Job drawing, mm, ordinate dimensions from the low corner. One solid piece. A direction names the side the tool comes from. Give positions to 0.01 mm unless a question says otherwise; leave off trailing zeros. Loops run counter-clockwise (first coordinate to the right, second up) from the corner with the lowest first, then second, coordinate; pieces in that order, holes last.
Item 1: Saw through at B-B on z = 1.5. Give the cut face in (x, y), plus the area to 3 significant figures.
Item 2: Mould opens along X. For the marked faces 5, 6, 7 and 8 say: released by +X, released by -X, zero draft, split by the parting line, or undercut.
Item 3: Drop flat-ended pins along their axis: P1, Ø0.8, axis at x = 12, z = 4, coming from the +Y side; P2, Ø8, axis at x = 8, y = 9, coming from the -Z side; P3, Ø0.5, axis at x = 12.5, y = 16, coming from the +Z side; P4, Ø4, axis at x = 7.5, y = 7.5, coming from the +Z side. Give the stop position or say it passes through.
Item 4: Saw through at A-A on x = 7.5. Give the cut face in (y, z).
Item 5: Probe probe 1 along Y at (x, z) = (7.5, 3.75); probe 2 along Z at (x, y) = (11.5, 6); probe 3 along Z at (x, y) = (11.5, 17.25). List the from-to ranges inside material, lowest first.
Item 6: Saw through at D-D on y = 13. Give the cut face in (x, z), plus the area to 3 significant figures.
Item 7: Which spindle directions (+Z, -Z, +X, -X, +Y, -Y) get a long thin tool onto all of the face, cutting with end or side? Do the marked faces 1, 2, 3 and 4. Say none if no direction does.
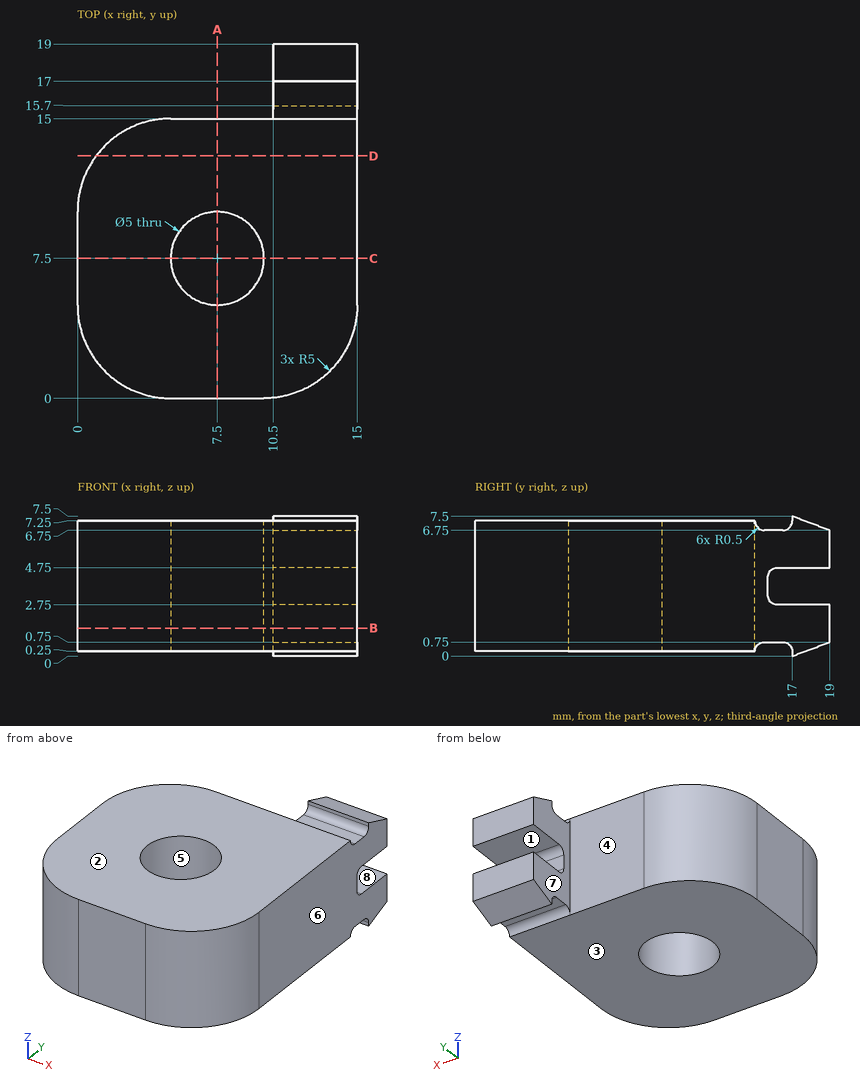
Results below:
1. outline: (0, 5) arc R5 ccw to (5, 0) - (10, 0) arc R5 ccw to (15, 5) - (15, 19) - (10.5, 19) - (10.5, 15) - (5, 15) arc R5 ccw to (0, 10) - close; hole circle Ø5 at (7.5, 7.5)
1. area: 207 mm2
2. face 5: undercut
2. face 6: released by +X
2. face 7: released by -X
2. face 8: zero draft
3. P1: stops at y = 15.72
3. P2: stops at z = 0.25
3. P3: stops at z = 6.75
3. P4: passes through
4. outline: (0, 0.25) - (5, 0.25) - (5, 7.25) - (0, 7.25) - close; (10, 0.25) - (15, 0.25) - (15, 7.25) - (10, 7.25) - close
5. probe 1: y = 0 to 5, 10 to 15
5. probe 2: z = 0.25 to 7.25
5. probe 3: z = 0.09 to 2.75, 4.75 to 7.41
6. outline: (1, 0.25) - (15, 0.25) - (15, 7.25) - (1, 7.25) - close
6. area: 98.0 mm2
7. face 1: +X, -X, +Y
7. face 2: +Z, +X, -X, -Y
7. face 3: -Z, +X, -X, -Y
7. face 4: +Z, -Z, -X, +Y
